```python
from build123d import *

# Parameters (mm, degrees)
CUT_EXTRUDE1_DEPTH      = 10
CUT_EXTRUDE1_DEPTH_BACK = 10
SKETCH7_W               = 161.67088451347962
SKETCH7_H               = 99.40268669666085
SKETCH8_W               = 4.999999999999993
SKETCH8_H               = 94
CUT_EXTRUDE2_DEPTH      = 35
SKETCH9_R               = 7.5
SKETCH9_R_2             = 4.000000000000013
SKETCH9_R_3             = 4.000000000000005
CUT_EXTRUDE3_DEPTH      = 405.82341829494015
SKETCH10_R              = 4.000000000000005
CUT_EXTRUDE4_DEPTH      = 433.4638713233743
SKETCH11_W              = 141.9999999999999
SKETCH11_H              = 16
BOSS_EXTRUDE1_DEPTH     = 380
FILLET2_R               = 5
FILLET3_R               = 5
FILLET4_R               = 5
FILLET5_R               = 5
FILLET6_R               = 5
CUT_EXTRUDE5_DEPTH      = 435.42030339292387


with BuildPart() as part:
    # Sweep2: sweep along a path in Sketch4
    with BuildLine(Plane.XY) as sweep2_path:
        Line((-65, 400), (-64.99999999999994, 10.000000000000007))
        ThreePointArc((-64.99999999999994, 10.000000000000007), (-62.07106781186544, 2.928932188134527), (-54.99999999999996, 0))
        Line((-54.99999999999996, 0), (54.99999999999999, 0))
        ThreePointArc((54.99999999999999, 0), (62.071067811865476, 2.9289321881345227), (65, 10))
        Line((65, 10), (65, 400))
        Line((65, 400), (-65, 400))
    # Sketch6 → Sweep2 (sweep)
    with BuildSketch(Plane(origin=(0, 0, 0), x_dir=(0, 0, -1), z_dir=(1, 0, 0))):
        Polygon((44.99999999999967, 406), (-45.00000000000032, 406), (-45.00000000000032, 393.99999999999994), (44.99999999999968, 394), align=None)
    sweep(path=sweep2_path.line, transition=Transition.RIGHT)

    # Sketch7 → Cut-Extrude1 (cut, two sides: drawn at the far end of the back side and taken through both)
    with BuildSketch(Plane(origin=(0, 0, 0), x_dir=(1, 0, 0), z_dir=(0, 1, 0)).offset(-CUT_EXTRUDE1_DEPTH_BACK)):
        Rectangle(SKETCH7_W, SKETCH7_H)
    extrude(amount=CUT_EXTRUDE1_DEPTH + CUT_EXTRUDE1_DEPTH_BACK, mode=Mode.SUBTRACT)

    # Sketch8 → Cut-Extrude2 (cut)
    with BuildSketch(Plane(origin=(0, 0, 0), x_dir=(1, 0, 0), z_dir=(0, 1, 0))):
        with Locations((-65.5, 0.24224418482823395)):
            Rectangle(SKETCH8_W, SKETCH8_H)
        with Locations((65.5, 0.24224418482823395)):
            Rectangle(SKETCH8_W, SKETCH8_H)
    extrude(amount=CUT_EXTRUDE2_DEPTH, mode=Mode.SUBTRACT)

    # Sketch9 → Cut-Extrude3 (cut, through all)
    with BuildSketch(Plane(origin=(0, 406, 0), x_dir=(1, 0, 0), z_dir=(0, 1, 0))):
        with Locations(Location((0, 0, 0), (0, 0, 270))):
            Circle(SKETCH9_R)
        with Locations(Location((-42, 31.999999999999993, 0), (0, 0, 270))):
            Circle(SKETCH9_R_2)
        with Locations(Location((-42, -32.00000000000001, 0), (0, 0, 270))):
            Circle(SKETCH9_R_3)
        with Locations(Location((42, -31.999999999999954, 0), (0, 0, 90))):
            Circle(SKETCH9_R_3)
        with Locations(Location((42, 32, 0), (0, 0, 90))):
            Circle(SKETCH9_R_2)
    extrude(amount=-CUT_EXTRUDE3_DEPTH, mode=Mode.SUBTRACT)

    # Sketch10 → Cut-Extrude4 (cut, through all)
    with BuildSketch(Plane(origin=(70.99999999999996, 0, 0), x_dir=(0, 0, -1), z_dir=(1, 0, 0))):
        with Locations((-37.999999999999936, 17.000000000000014)):
            Circle(SKETCH10_R)
    extrude(amount=-CUT_EXTRUDE4_DEPTH, mode=Mode.SUBTRACT)

    # Sketch11 → Boss-Extrude1 (add)
    with BuildSketch(Plane(origin=(0, 406, 0), x_dir=(1, 0, 0), z_dir=(0, 1, 0))):
        with Locations((0, -52.999999999999936)):
            Rectangle(SKETCH11_W, SKETCH11_H)
    extrude(amount=-BOSS_EXTRUDE1_DEPTH)

    # Fillet2
    fillet2_edges = [part.edges().sort_by_distance(p)[0] for p in [
        (59.00000000000001, 202, -44.99999999999968),
    ]]
    fillet(fillet2_edges, radius=FILLET2_R)

    # Fillet3
    fillet3_edges = [part.edges().sort_by_distance(p)[0] for p in [
        (71, 208, -44.99999999999967),
    ]]
    fillet(fillet3_edges, radius=FILLET3_R)

    # Fillet4
    fillet4_edges = [part.edges().sort_by_distance(p)[0] for p in [
        (-59.00000000000001, 202, -44.99999999999968),
    ]]
    fillet(fillet4_edges, radius=FILLET4_R)

    # Fillet5
    fillet5_edges = [part.edges().sort_by_distance(p)[0] for p in [
        (-71, 208, -44.99999999999967),
    ]]
    fillet(fillet5_edges, radius=FILLET5_R)

    # Fillet6
    fillet6_edges = [part.edges().sort_by_distance(p)[0] for p in [
        (70.99999999999994, 216, 60.999999999999936),
        (-70.99999999999994, 216, 60.999999999999936),
        (0, 406, 60.999999999999936),
        (0, 406, -44.99999999999967),
        (0, 406, -44.99999999999967),
        (70.99999999999997, 406, 10.500000000000085),
        (-70.99999999999997, 406, 10.500000000000135),
        (69.53553390593274, 406, -43.53553390593251),
        (-69.53553390593274, 406, -43.53553390593241),
    ]]
    fillet(fillet6_edges, radius=FILLET6_R)

    # Sketch12 → Cut-Extrude5 (cut, through all)
    with BuildSketch(Plane.ZY.offset(70.9999999999999)):
        with BuildLine():
            Line((-19.99811023879916, 9.999999999999995), (-79.77303285275339, 10.000000000000018))
            Line((-79.77303285275339, 10.000000000000018), (-79.77303285275339, 406.4421165391139))
            Line((-79.77303285275339, 406.4421165391139), (-17.24924979661946, 406))
            ThreePointArc((-17.24924979661946, 406), (-27.67595887590869, 208.0628369981441), (-19.99811023879916, 9.999999999999995))
        make_face()
    extrude(amount=-CUT_EXTRUDE5_DEPTH, mode=Mode.SUBTRACT)


solid = part.part
```
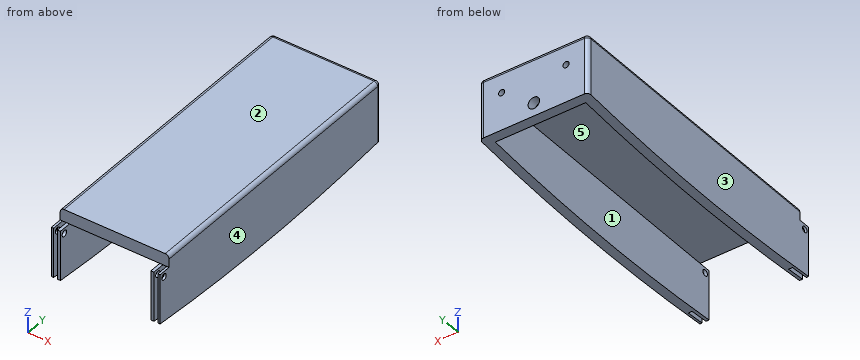
Check sheet for the modelled part. Datum: model origin and axes. Units: mm. Face numbers are marked on the shaded views. A direction names the side the tool comes from. Round coordinates to 2 decimals unless told otherwise and drop trailing zeros. Loops run counter-clockwise (first coordinate to the right, second up) from the corner with the lowest first, then second, coordinate; pieces in that order, holes last. Notation, with made-up numbers: (64.5, 78) -> (85.5, 78) arc R11 cw to (85.5, 93) -> close; hole circle Ø5 at (79.25, 85). An arc over 180 degrees is marked (long way). Write item = value, one per line. Start each with the question number.
1) Gauge pin test, flat ends, axial feed: pin 1 Ø2 at (x, z) = (-20.5, -14.5) entering from -Y; pin 2 Ø1 at (x, y) = (8, 131) entering from -Z; pin 3 Ø2.5 at (x, y) = (-70, 15) entering from +Z; pin 4 Ø10.5 at (y, z) = (17, 38) entering from +X. Record the tip position at first contact, or that the pin passes through.
2) Thickness scan on probe 1 along X at (y, z) = (401.25, 32); probe 2 along X at (y, z) = (399, 0); probe 3 along X at (y, z) = (304, 14.5). Record the ranges inside material, lowest first.
3) Set-up check for the marked faces 1 and 2: record each of +Z, -Z, +X, -X, +Y, -Y from which the full face is reachable in a straight line by a thin tool's end or side.
4) Sectioned sample at B-B, the plane y = 17. State how many separate pieces and enclosed holes the cut face has, plus the area to 3 significant figures.
5) Release check for a two-part mould opening along X. For the marked faces 3, 4 and 5 record: released by +X, released by -X, zero draft, split by the parting line, or undercut.
6) Sectioned sample at C-C, the plane z = -2. Record the cut outline in (x, y), plus the area to 3 significant figures.
7) Sectioned sample at D-D, the plane x = -42. Record the cut outline in (y, z), plus the area to 3 significant figures.
8) Sectioned sample at A-A, the plane x = 0. Record the cut outline in (y, z), plus the area to 3 significant figures.
Results are:
q1.pin_1 = 394
q1.pin_2 = 45
q1.pin_3 = 45
q1.pin_4 = 71
q2.probe_1 = -70.99 to -46, -38 to 38, 46 to 70.99
q2.probe_2 = -71 to -7.5, 7.5 to 71
q2.probe_3 = -71 to -59, 59 to 71
q3.face_1 = -Z, -Y
q3.face_2 = +Z, +X, -X, +Y, -Y
q4.separate_pieces = 8
q4.enclosed_holes = 0
q4.area = 806 mm^2
q5.face_3 = released by -X
q5.face_4 = released by +X
q5.face_5 = undercut
q6.outline = (-71, 10) -> (-68, 10) -> (-68, 35) -> (-63, 35) -> (-63, 10) -> (-59, 10) -> (-59, 394) -> (-7.23, 394) -> (-7.23, 406) -> (-66, 406) arc R5 ccw to (-71, 401) -> close; (7.23, 394) -> (59, 394) -> (59, 10) -> (63, 10) -> (63, 35) -> (68, 35) -> (68, 10) -> (71, 10) -> (71, 401) arc R5 ccw to (66, 406) -> (7.23, 406) -> close
q6.area = 10,500 mm^2
q7.outline = (26, 45) -> (394, 45) -> (394, 36) -> (406, 36) -> (406, 56) arc R5 ccw to (401, 61) -> (26, 61) -> close; (394, -18.4) arc R2170 ccw to (406, -17.25) -> (406, 28) -> (394, 28) -> close
q7.area = 6,730 mm^2
q8.outline = (26, 45) -> (394, 45) -> (394, 7.5) -> (406, 7.5) -> (406, 56) arc R5 ccw to (401, 61) -> (26, 61) -> close; (394, -18.4) arc R2170 ccw to (406, -17.25) -> (406, -7.5) -> (394, -7.5) -> close
q8.area = 6,650 mm^2
